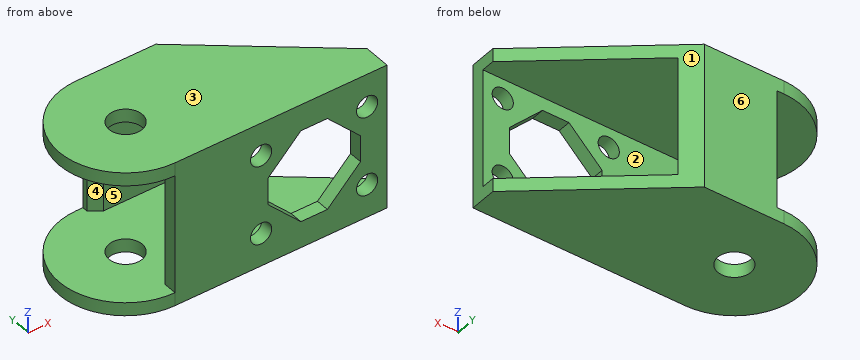
Autodesk Inventor part; units mm, degrees
ref_plane "Work Plane1" through (0, 0, -9) normal (0, 0, -1) x (-1, 0, 0)
ref_plane "YZ Plane" through (0, 0, 0) normal (1, 0, 0) x (0, 1, 0)
ref_plane "XZ Plane" through (0, 0, 0) normal (0, 1, 0) x (-1, 0, 0)
sketch "Sketch1" plane through (0, 0, 0) normal (0, 0, 1) x (1, 0, 0)
  circle A0 centre (0, 0) radius 2.5
  arc A1 (0, 10) -> (0, -10) centre (0, 0) ccw
  line L0 (0, 10) -> (12, 10)
  line L1 (0, -10) -> (12, -10)
  line L2 (12, -10) -> (12, 10)
  dimension "d0" = 5
  dimension "d1" = 20
  dimension "d2" = 12
extrude "Extrusion1" add sketch "Sketch1" along normal blind 2
sketch "Sketch5" plane through (0, 0, 0) normal (0, 0, -1) x (-1, 0, 0)
  circle A0 centre (0, 0) radius 2.5
  line L0 (-12, -10) -> (0, -10)
  line L1 (0, -10) -> (0, -8)
  line L2 (0, -8) -> (-12, -8)
  line L3 (-12, -8) -> (-12, -10)
  line L4 (-12, 10) -> (-1, 10)
  line L5 (-1, 10) -> (-1, 8)
  line L6 (-1, 8) -> (-12, 8)
  line L7 (-12, 8) -> (-12, 10)
  dimension "d21" = 2
  dimension "d22" = 2
  dimension "d24" = 1
extrude "Extrusion5" add sketch "Sketch5" along normal blind 2 contours L3 L2 L1 L0 | L4 L5 L6 L7
sketch "Sketch6" plane through (0, 0, -2) normal (0, 0, -1) x (-1, 0, 0)
  line L0 (-12, 8) -> (-1, 8)
  line L1 (-1, 8) -> (-1, 10)
  line L2 (-1, 9.162) -> (-2.5994, 8)
  line L3 (-2.5994, 8) -> (6.8052, -4.9443) construction
  line L4 (6.8052, -4.9443) -> (8.4046, -3.7823) construction
  line L5 (8.4046, -3.7823) -> (-1, 9.162) construction
  line L6 (-2.5994, 8) -> (-1, 8)
  line L7 (-1, 9.162) -> (-1, 8)
  point P0 (0, 0)
  dimension "d27" = 16
  dimension "d28" = 8
  dimension "d29" = 36
extrude "Extrusion6" cut sketch "Sketch6" against normal blind 2
ref_plane "Work Plane1" through (0, 0, -9) normal (0, 0, -1) x (-1, 0, 0)
mirror "Mirror1" about plane through (0, 0, -9) normal (0, 0, -1)
sketch "Sketch7" plane through (0, -10, -16) normal (0, 0, 1) x (1, 0, 0)
  line L0 (12, 0) -> (0, 0)
  line L1 (12, 2) -> (12, 0)
  line L2 (0, 2) -> (12, 2)
  line L3 (0, 0) -> (0, 2)
  line L4 (2.5994, 18) -> (1, 19.162)
  line L5 (12, 18) -> (2.5994, 18)
  line L6 (12, 20) -> (12, 18)
  line L7 (1, 20) -> (12, 20)
  line L8 (1, 19.162) -> (1, 20)
  point P0 (0, 10)
extrude "Extrusion7" add sketch "Sketch7" along normal blind 14
sketch "Sketch8" plane through (12, -10, 2) normal (1, 0, 0) x (0, 0, -1)
  line L0 (22, 20) -> (0, 20)
  line L1 (0, 0) -> (0, 20)
  line L2 (22, 0) -> (0, 0)
  line L3 (22, 0) -> (22, 20)
  line L4 (2, 18) -> (20, 18)
  line L5 (20, 2) -> (20, 18)
  line L6 (2, 2) -> (20, 2)
  line L7 (2, 2) -> (2, 18)
  point P0 (2, 10)
extrude "Extrusion8" add sketch "Sketch8" along normal blind 20
sketch "Sketch9" plane through (0, 0, -20) normal (0, 0, -1) x (-1, 0, 0)
  line L0 (-32, 10) -> (0, 10)
  line L1 (-32, -10) -> (-32, 10)
  line L2 (-32, -6) -> (-12, 10)
  dimension "d37" = 20
  dimension "d38" = 4
extrude "Extrusion9" cut sketch "Sketch9" against normal blind 22
sketch "Sketch10" plane through (0, -8, 0) normal (0, 1, 0) x (1, 0, 0)
  line L0 (32, 0) -> (0, 0)
  line L1 (32, 18) -> (32, 0)
  line L2 (0, 18) -> (32, 18)
  line L3 (13, 15) -> (29, 15) construction
  line L4 (29, 15) -> (29, 3) construction
  line L5 (29, 3) -> (13, 3) construction
  line L6 (13, 3) -> (13, 15) construction
  circle A0 centre (13, 15) radius 1.6
  circle A1 centre (29, 15) radius 1.6
  circle A2 centre (29, 3) radius 1.6
  circle A3 centre (13, 3) radius 1.6
  line L7 (19, 16) -> (23, 16)
  line L8 (28, 11) -> (28, 7)
  line L9 (23, 2) -> (19, 2)
  line L10 (14, 7) -> (14, 11)
  line L11 (14, 7) -> (19, 2)
  line L12 (23, 2) -> (28, 7)
  line L13 (28, 11) -> (23, 16)
  line L14 (19, 16) -> (14, 11)
  point P0 (14, 9)
  point P1 (13, 9)
  dimension "d41" = 3.2
  dimension "d42" = 3
  dimension "d43" = 3
  dimension "d44" = 3
  dimension "d45" = 16
  dimension "d46" = 45
  dimension "d47" = 4
  dimension "d48" = 1
  dimension "d49" = 1
extrude "Extrusion10" cut sketch "Sketch10" against normal through all
properties part number "z_axis_cable_mount_a" material "ABS Plastic"
Here's how the part is built. I have some questions about the finished solid (model axes, mm). Face numbers are marked on the shaded views. A direction names the side the tool comes from. Coordinates: 2 decimals unless noted, no trailing zeros. Order: outer loops, then holes, each group sorted by start corner. A loop starts at its lowest first (then second) coordinate and runs counter-clockwise, first axis right, second up. Notation, with made-up numbers: (23, 80.5) -> (35, 80.5) arc R18 cw to (35, 93.5) -> close; hole circle Ø9 at (-10.5, 78.25). An arc over 180 degrees is marked (long way). Return JSON: item names as keys, results as strings.
1) If we section it at B-B on y = 6: List the corners of the cut face in (x, z) for me.
Conclusion:
{"outline": "(-8, -20) -> (17, -20) -> (17, -18) -> (-8, -18) -> close; (-8, 0) -> (17, 0) -> (17, 2) -> (-8, 2) -> close"}
2) If we section it at A-A on x = 24.5: List the corners of the cut face in (y, z) for me, plus the area to 3 significant figures.
Conclusion:
{"outline": "(-10, -20) -> (0, -20) -> (0, -18) -> (-8, -18) -> (-8, -14.5) -> (-10, -14.5) -> close; (-10, -3.5) -> (-8, -3.5) -> (-8, 0) -> (0, 0) -> (0, 2) -> (-10, 2) -> close", "area": "54.0 mm²"}
3) If we section it at D-D on z = -15: List the corners of the cut face in (x, y) for me, plus the area to 3 significant figures.
Conclusion:
{"outline": "(0, -10) -> (11.4, -10) -> (11.4, -8) -> (0, -8) -> close; (1, 9.16) -> (2.6, 8) -> (14.5, 8) -> (12, 10) -> (1, 10) -> close; (14.6, -10) -> (18, -10) -> (18, -8) -> (14.6, -8) -> close; (24, -10) -> (27.4, -10) -> (27.4, -8) -> (24, -8) -> close; (30.6, -10) -> (32, -10) -> (32, -8) -> (30.6, -8) -> close", "area": "62.8 mm²"}
4) If I drill on probe 1 along Z at (x, y) = (13, -8.7); probe 2 along Z at (x, y) = (11, -4); probe 3 along Y at (x, z) = (0, 1.2), over which ranges is the centre line in solid material (lowest first)?
Conclusion:
{"probe 1": "z = -20 to -16.6, -13.4 to -4.6, -1.4 to 2", "probe 2": "z = -20 to -18, 0 to 2", "probe 3": "y = -10 to -2.5, 2.5 to 10"}
5) If we section it at C-C on z = -12.25: List the corners of the cut face in (x, y) for me.
Conclusion:
{"outline": "(0, -10) -> (15.25, -10) -> (15.25, -8) -> (0, -8) -> close; (1, 9.16) -> (2.6, 8) -> (14.5, 8) -> (12, 10) -> (1, 10) -> close; (26.75, -10) -> (32, -10) -> (32, -8) -> (26.75, -8) -> close"}
6) I'm going to push flat-ended pins straight in: P1, Ø1.9, axis at x = 13, z = -15, coming from the -Y side; P2, Ø8, axis at y = 3.5, z = -15, coming from the +X side; P3, Ø1.6, axis at y = -9, z = -4.5, coming from the -X side. Where does each tip first touch, or does it pass through?
Conclusion:
{"P1": "stops at y = 8", "P2": "stops at x = 23.43", "P3": "stops at x = 0"}
7) On a 3-axis mill with a long thin cutter (end or side, diameter ignored), from which of +Z, -Z, +X, -X, +Y, -Y can I reach the whole of each face in a straight line? I mean the marked faces 4, 5 and 6. Say none if no direction works.
Conclusion:
{"face 4": "-X", "face 5": "+X, -X", "face 6": "+Z, -Z, +X, -X, +Y"}
8) Thinking about a two-plate mould opening in Z: for the marked faces 1, 2 and 3, which applies, +Z half, -Z half, draft (parallel to the pull), parting line (faces both ways), or undercut?
Conclusion:
{"face 1": "draft", "face 2": "undercut", "face 3": "+Z half"}
